```python
from build123d import *

# Parameters (mm, degrees)
EXTRUDE_1_DEPTH          = 30
EXTRUDE_1_DEPTH_BACK     = 30
SKETCH_2_W               = 30
SKETCH_2_H               = 40
CUT_EXTRUDE_1_DEPTH      = 32
SKETCH_3_W               = 10
SKETCH_3_H               = 10
CUT_EXTRUDE_2_DEPTH      = 61
SKETCH_4_R               = 14.906957443
EXTRUDE_2_DEPTH          = 15
CUT_EXTRUDE_3_DEPTH      = 37
CUT_EXTRUDE_3_DEPTH_BACK = 26
EXTRUDE_3_DEPTH          = 4
EXTRUDE_3_DEPTH_BACK     = 4
EXTRUDE_4_DEPTH          = 4
EXTRUDE_4_DEPTH_BACK     = 4


with BuildPart() as part:
    # Эскиз1 → Бобышка-Вытянуть1 (new body, two sides)
    with BuildSketch(Plane.XY) as extrude_1_sk:
        Polygon((0, 0), (80, 0), (80, 45), (65, 65.371127092), (65, 103.371127092), (40, 103.371127092), (15, 103.371127092), (15, 65.371127092), (0, 45), align=None)
        Polygon((10, 10), (70, 10), (70, 41.715496922), (60.218138384, 55), (19.781861616, 55), (10, 41.715496922), align=None, mode=Mode.SUBTRACT)
    extrude(amount=EXTRUDE_1_DEPTH)
    extrude(extrude_1_sk.sketch, amount=-EXTRUDE_1_DEPTH_BACK)

    # Эскиз2 → Вырез-Вытянуть1 (cut)
    with BuildSketch(Plane(origin=(0, 103.371127092, 0), x_dir=(1, 0, 0), z_dir=(0, 1, 0))):
        with Locations((39.906957443, -0.006497208)):
            Rectangle(SKETCH_2_W, SKETCH_2_H)
    extrude(amount=-CUT_EXTRUDE_1_DEPTH, mode=Mode.SUBTRACT)

    # Эскиз3 → Вырез-Вытянуть2 (cut, through all)
    with BuildSketch(Plane.XY.offset(30)):
        with Locations((40, 103.371127092)):
            Rectangle(SKETCH_3_W, SKETCH_3_H)
    extrude(amount=-CUT_EXTRUDE_2_DEPTH, mode=Mode.SUBTRACT)

    # Эскиз4 → Бобышка-Вытянуть2 (add)
    with BuildSketch(Plane(origin=(0, 10, 0), x_dir=(1, 0, 0), z_dir=(0, 1, 0))):
        with Locations((40, 0)):
            Circle(SKETCH_4_R)
    extrude(amount=EXTRUDE_2_DEPTH)

    # Эскиз5 → Вырез-Вытянуть3 (cut, two sides)
    with BuildSketch(Plane(origin=(0, 25, 0), x_dir=(1, 0, 0), z_dir=(0, 1, 0))) as cut_extrude_3_sk:
        Polygon((40, 9.192388155), (30.807611845, 0), (40, -9.192388155), (49.192388155, 0), align=None)
    extrude(amount=CUT_EXTRUDE_3_DEPTH, mode=Mode.SUBTRACT)
    extrude(cut_extrude_3_sk.sketch, amount=-CUT_EXTRUDE_3_DEPTH_BACK, mode=Mode.SUBTRACT)

    # Эскиз6 → Бобышка-Вытянуть3 (add, two sides)
    with BuildSketch(Plane.XY) as extrude_3_sk:
        Polygon((70, 10), (51.541791272, 10), (51.541791272, 20.404686065), (70, 41.715496922), align=None)
        Polygon((10, 10), (10, 41.715496922), (28.458208728, 20.404686065), (28.458208728, 10), align=None)
    extrude(amount=EXTRUDE_3_DEPTH)
    extrude(extrude_3_sk.sketch, amount=-EXTRUDE_3_DEPTH_BACK)

    # Эскиз8 → Бобышка-Вытянуть4 (add, two sides)
    with BuildSketch(Plane.XY) as extrude_4_sk:
        with BuildLine():
            Line((54.906957443, 103.371127092), (54.906957443, 77.371127092))
            Line((54.906957443, 77.371127092), (54.906957443, 71.371127092))
            Line((54.906957443, 71.371127092), (24.906957443, 71.371127092))
            Line((24.906957443, 71.371127092), (24.906957443, 77.371127092))
            Line((24.906957443, 77.371127092), (24.906957443, 103.371127092))
            add(Edge.make_bspline(
                [(24.906957443, 103.371127092), (39.906957443, 51.371127092), (54.906957443, 103.371127092)],
                knots=[0, 0, 0, 1, 1, 1], degree=2))
        make_face()
    extrude(amount=EXTRUDE_4_DEPTH)
    extrude(extrude_4_sk.sketch, amount=-EXTRUDE_4_DEPTH_BACK)


solid = part.part
```
Work out the finished part from the listing and answer in its coordinate system (mm). A direction names the side the tool comes from. Give positions to 0.01 mm unless a question says otherwise; leave off trailing zeros. Loops run counter-clockwise (first coordinate to the right, second up) from the corner with the lowest first, then second, coordinate; pieces in that order, holes last. Notation, with made-up numbers: (-28, 38.25) -> (16, 38.25) arc R14 cw to (16, 42.25) -> close; hole circle Ø11 at (25.25, 61.25). An arc over 180 degrees is marked (long way). Use CSV: the item, a comma, the result in double quotes.
1. The part is cut by section A-A (z = -25). Write down the section's boundary in (x, y), then the cut area to 3 significant figures.
Found:
outline,"(0, 0) -> (80, 0) -> (80, 45) -> (65, 65.37) -> (65, 103.37) -> (45, 103.37) -> (45, 98.37) -> (35, 98.37) -> (35, 103.37) -> (15, 103.37) -> (15, 65.37) -> (0, 45) -> close; hole (10, 10) -> (70, 10) -> (70, 41.72) -> (60.22, 55) -> (19.78, 55) -> (10, 41.72) -> close"
area,"4,200 mm^2"
2. The mould has two halves that part along Z. Classify faces 6 (the flat face through (39, 64, -30)), 7 (the flat face through (40, 88, 20.006)), 8 (the flat face through (39, 77, -4)), 9 (the flat face through (70, 26, -17)): +Z half, -Z half, draft (parallel to the pull), parting line (faces both ways), or undercut.
Found:
face 6,"-Z half"
face 7,"undercut"
face 8,"undercut"
face 9,"draft"
3. The part is cut by section C-C (y = 59.5). Write down the section's boundary in (x, z).
Found:
outline,"(10.68, -30) -> (69.32, -30) -> (69.32, 30) -> (10.68, 30) -> close; hole (30.81, 0) -> (40, -9.19) -> (49.19, 0) -> (40, 9.19) -> close"
4. A tool of negligible diameter and unlimited length cuts with its end or side. For faces 1 (the flat face through (64, 23, -4)), 2 (the flat face through (40, 62, 0)), 3 (the flat face through (54.907, 88, 12)), 4 (the flat face through (65.18, 48.26, 0.42)), 5 (the flat face through (10, 26, 17)), from which of +Z, -Z, +X, -X, +Y, -Y can it reach the whole face along a straight path? Write none if from no direction.
Found:
face 1,"-Z"
face 2,"-Y"
face 3,"+Y"
face 4,"+Z, -Z"
face 5,"+Z"
5. The part is cut by section B-B (y = 27). Write down the section's boundary in (x, z).
Found:
outline,"(0, -30) -> (10, -30) -> (10, -4) -> (22.75, -4) -> (22.75, 4) -> (10, 4) -> (10, 30) -> (0, 30) -> close; (57.25, -4) -> (70, -4) -> (70, -30) -> (80, -30) -> (80, 30) -> (70, 30) -> (70, 4) -> (57.25, 4) -> close"
6. Straight lines are drawn through the part: line 1 (Z direction, x = 53, y = 80); line 2 (X direction, y = 31.5, z = -7); line 3 (X direction, y = 83, z = 9). For each, find the intervals that lie inside material, in ascending order.
Found:
line 1,"-30 to -19.99, -4 to 4, 20.01 to 30"
line 2,"0 to 10, 70 to 80"
line 3,"15 to 24.91, 54.91 to 65"
7. The part is cut by section D-D (z = -11.5). Write down the section's boundary in (x, y), then the cut area to 3 significant figures.
Found:
outline,"(0, 0) -> (80, 0) -> (80, 45) -> (65, 65.37) -> (65, 103.37) -> (54.91, 103.37) -> (54.91, 71.37) -> (24.91, 71.37) -> (24.91, 103.37) -> (15, 103.37) -> (15, 65.37) -> (0, 45) -> close; hole (10, 10) -> (30.51, 10) -> (30.51, 25) -> (49.49, 25) -> (49.49, 10) -> (70, 10) -> (70, 41.72) -> (60.22, 55) -> (19.78, 55) -> (10, 41.72) -> close"
area,"3,580 mm^2"
8. Flat-ended cylindrical pins translate along their axes: pin 1 Ø12.5 at (x, y) = (63.5, 31) entering from -Z; pin 2 Ø8 at (x, z) = (66.5, -5.5) entering from -Y; pin 3 Ø5 at (y, z) = (86.5, -14.5) entering from +X; pin 4 Ø13 at (y, z) = (79.5, -10) entering from -X. Find the tip coordinate at first contact, or state that the pin passes through.
Found:
pin 1,"z = -4"
pin 2,"y = 0"
pin 3,"x = 65"
pin 4,"x = 15"
